Build history of the part. All positions in model axes, mm. Give positions to 0.01 mm unless a question says otherwise; leave off trailing zeros. Write each loop counter-clockwise with the first axis right and the second up, starting at its lowest first coordinate (ties: lowest second). Pieces come first, ordered by that corner, then holes. Notation, with made-up numbers: (13.25, 85) - (69.25, 85) arc R10 ccw to (69.25, 102) - close; hole circle Ø10 at (-9, 52.5). An arc over 180 degrees is marked (long way). Use one line per item in the form item = value. Start each with the question number.
Autodesk Inventor part; units mm, degrees
ref_plane "YZ Plane" through (0, 0, 0) normal (1, 0, 0) x (0, 1, 0)
ref_plane "XZ Plane" through (0, 0, 0) normal (0, 1, 0) x (-1, 0, 0)
ref_plane "XY Plane" through (0, 0, 0) normal (0, 0, 1) x (1, 0, 0)
sketch "草圖1" plane through (0, 0, 0) normal (0, 0, 1) x (1, 0, 0)
  circle A0 centre (0, 0) radius 22.5
  circle A1 centre (0, 0) radius 31
  dimension "d0" = 45
  dimension "d1" = 62
extrude "擠出1" add sketch "草圖1" along normal blind 0.8
sketch "草圖2" plane through (0, 0, 0.8) normal (0, 0, 1) x (1, 0, 0)
  line L0 (-6.1, 25.6) -> (6.1, 25.6)
  line L1 (6.1, 25.6) -> (6.1, 13.8504)
  line L2 (6.1, 13.8504) -> (-6.1, 13.8504)
  line L3 (-6.1, 13.8504) -> (-6.1, 25.6)
  point P0 (0, 0)
  dimension "d5" = 6.1
  dimension "d6" = 12.2
  dimension "d7" = 25.6
extrude "擠出2" cut sketch "草圖2" against normal blind 0.8
properties part number "軸心墊片"
(1) Cut at C-C, the plane y = 0. Give the cut face in (x, z).
(2) Two-plate mould, pull along X, no slides. Class faces 1 (the flat face through (9, 21, 0)), 2 (the cylindrical face through (0.9, -22.48, 0.39)), 3 (the cylindrical face through (-4.036, -30.736, 0.394)): +X half, -X half, draft (parallel to the pull), parting line (faces both ways), or undercut.
(3) Cut at B-B, the plane z = 0.6. Give the cut face in (x, y), then the cut area to 3 significant figures.
(4) Wall check: line 1 (Y direction, x = 0, z = 0.25); line 2 (Y direction, x = -18.5, z = 0.2); line 3 (X direction, y = 4, z = 0.25). Give the ranges that are in metal, low to high. Write a range as from..to.
(5) Cut at A-A, the plane x = 0. Give the cut face in (y, z), then the cut area to 3 significant figures.
(6) Cut at D-D, the plane x = 27. Give the cut face in (y, z), then the cut area to 3 significant figures.
Solution:
q1.outline = (-31, 0) - (-22.5, 0) - (-22.5, 0.8) - (-31, 0.8) - close; (22.5, 0) - (31, 0) - (31, 0.8) - (22.5, 0.8) - close
q2.face_1 = draft
q2.face_2 = undercut
q2.face_3 = parting line
q3.outline = circle Ø62 at (0, 0); hole (-6.1, 21.66) arc R22.5 ccw (long way) to (6.1, 21.66) - (6.1, 25.6) - (-6.1, 25.6) - close
q3.area = 1,390 mm2
q4.line_1 = -31..-22.5, 25.6..31
q4.line_2 = -24.87..-12.81, 12.81..24.87
q4.line_3 = -30.74..-22.14, 22.14..30.74
q5.outline = (-31, 0) - (-22.5, 0) - (-22.5, 0.8) - (-31, 0.8) - close; (25.6, 0) - (31, 0) - (31, 0.8) - (25.6, 0.8) - close
q5.area = 11.1 mm2
q6.outline = (-15.23, 0) - (15.23, 0) - (15.23, 0.8) - (-15.23, 0.8) - close
q6.area = 24.4 mm2
